```python
from build123d import *

# Parameters (mm, degrees)
ESBO_O1_R                                   = 12.2
RESSALTO_EXTRUS_O1_DEPTH                    = 40
ESBO_O2_R                                   = 3.2
RESSALTO_EXTRUS_O2_DEPTH                    = 1.7
ESBO_O3_R                                   = 1
RESSALTO_EXTRUS_O3_DEPTH                    = 5.3
BROCA_DE_ROSQUEAR_PARA_TARRAXA_DE_M31_D     = 2.5
BROCA_DE_ROSQUEAR_PARA_TARRAXA_DE_M31_DEPTH = 4
BROCA_DE_ROSQUEAR_PARA_TARRAXA_DE_M31_TIP   = 0.751075774
FILETE1_R                                   = 1
FILETE2_R                                   = 1


with BuildPart() as part:
    # Esboço1 → Ressalto-extrusão1 (new body)
    with BuildSketch(Plane.XY):
        Circle(ESBO_O1_R)
    extrude(amount=RESSALTO_EXTRUS_O1_DEPTH)

    # Esboço2 → Ressalto-extrusão2 (add)
    with BuildSketch(Plane.XY.offset(40)):
        Circle(ESBO_O2_R)
    extrude(amount=RESSALTO_EXTRUS_O2_DEPTH)

    # Esboço3 → Ressalto-extrusão3 (add)
    with BuildSketch(Plane.XY.offset(41.7)):
        Circle(ESBO_O3_R)
    extrude(amount=RESSALTO_EXTRUS_O3_DEPTH)

    # Broca de rosquear para tarraxa de M31
    with Locations(Plane(origin=(-8.6, 0, 40), x_dir=(1, 0, 0), z_dir=(0, 0, 1))):
        with Locations((0, 0), (17.2, 0)):
            Hole(BROCA_DE_ROSQUEAR_PARA_TARRAXA_DE_M31_D / 2, depth=BROCA_DE_ROSQUEAR_PARA_TARRAXA_DE_M31_DEPTH)
            with Locations((0, 0, -(BROCA_DE_ROSQUEAR_PARA_TARRAXA_DE_M31_DEPTH + BROCA_DE_ROSQUEAR_PARA_TARRAXA_DE_M31_TIP / 2))):  # 118° drill point
                Cone(0, BROCA_DE_ROSQUEAR_PARA_TARRAXA_DE_M31_D / 2, BROCA_DE_ROSQUEAR_PARA_TARRAXA_DE_M31_TIP, mode=Mode.SUBTRACT)

    # Filete1
    filete1_edges = [part.edges().sort_by_distance(p)[0] for p in [
        (-12.2, 0, 40),
    ]]
    fillet(filete1_edges, radius=FILETE1_R)

    # Filete2
    filete2_edges = [part.edges().sort_by_distance(p)[0] for p in [
        (-12.2, 0, 0),
    ]]
    fillet(filete2_edges, radius=FILETE2_R)


solid = part.part
```
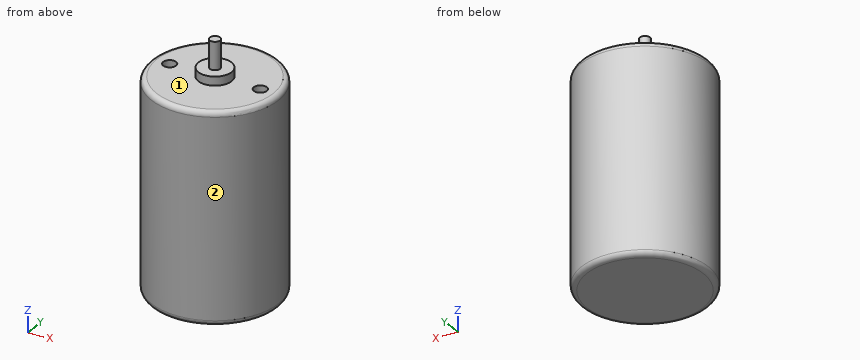
Input: part model. Units: mm. Frame: model coordinates. Face numbers are marked on the shaded views. A direction names the side the tool comes from. Coordinates: 2 decimals unless noted, no trailing zeros. Loops run counter-clockwise (first coordinate to the right, second up) from the corner with the lowest first, then second, coordinate; pieces in that order, holes last. Notation, with made-up numbers: M 13,-5 L 22,-5 A10 ccw 22,-1 Z; hole C 81.5,76.5 d8. An arc over 180 degrees is marked long. Answer in a Markdown table with one row per item.
1. Section A-A, the plane x = 0. Output: boundary loops of the cut face in (y, z), then the cut area to 3 significant figures.
Response:
| item | result |
|---|---|
| outline | M -12.2,1 A1 ccw -11.2,0 L 11.2,0 A1 ccw 12.2,1 L 12.2,39 A1 ccw 11.2,40 L 3.2,40 L 3.2,41.7 L 1,41.7 L 1,47 L -1,47 L -1,41.7 L -3.2,41.7 L -3.2,40 L -11.2,40 A1 ccw -12.2,39 Z |
| area | 997 mm2 |
2. First-contact query: pin 1 (1.5 mm diameter, centred on x = 8.5, z = 7, fed in from -Y); pin 2 (4 mm diameter, centred on x = -8.5, z = 22, fed in from -Y); pin 3 (1.5 mm diameter, centred on y = 6.5, z = 35, fed in from +X). Flat tips, straight axial feed; report the tip coordinate or a pass-through.
Response:
| item | result |
|---|---|
| pin 1 | stops at y = -9.42 |
| pin 2 | stops at y = -10.32 |
| pin 3 | stops at x = 10.76 |
3. Material intervals for line 1 (Y direction, x = -0.25, z = 9.5); line 2 (Z direction, x = 1.5, y = -8.75); line 3 (Z direction, x = -0.5, y = 2), sorted ascending.
Response:
| item | result |
|---|---|
| line 1 | y = -12.2 to 12.2 |
| line 2 | z = 0 to 40 |
| line 3 | z = 0 to 41.7 |
4. Section B-B, the plane z = 19. Output: boundary loops of the cut face in (x, y).
Response:
| item | result |
|---|---|
| outline | C 0,0 d24.4 |
5. Reachability of the marked faces 1 and 2 from +Z, -Z, +X, -X, +Y, -Y: full face, straight path, thin tool, end or side. Return the list, or none.
Response:
| item | result |
|---|---|
| face 1 | +Z |
| face 2 | +Z, -Z |
